Here's how the part is built. I have some questions about the finished solid (model axes, mm). A direction names the side the tool comes from. Round coordinates to 2 decimals unless told otherwise and drop trailing zeros. Write each loop counter-clockwise with the first axis right and the second up, starting at its lowest first coordinate (ties: lowest second). Pieces come first, ordered by that corner, then holes. Notation, with made-up numbers: (22.5, 2) - (45.5, 2) arc R35 cw to (45.5, 34) - close; hole circle Ø7 at (-6, 67). An arc over 180 degrees is marked (long way). Write item = value, one per line. Start each with the question number.
Item 1: Thinking about a two-plate mould opening in Y: for faces 3 (the face through (58.681, 294, 1)), 4 (the face through (21, 295.136, 1)), 5 (the face through (7.682, 293.538, 1.479)), 6 (the face through (35, 294, 0)), which applies, pulls with the +Y half, pulls with the -Y half, needs draft (parallel to the pull), parting line crosses it, or undercut?
Item 2: If we section it at B-B (z = 2.45): Please give me the cut outline in (x, y).
Item 3: If we section it at A-A (y = 294): Please give me the cut outline in (x, z), and give its area (3 significant figures).
Item 4: Which directions (+Z, -Z, +X, -X, +Y, -Y) give clear straight access to the entire face, cutting with the end or side of a thin tool? Please do faces 1 (the face through (35, 294, 3)), 2 (the face through (19.681, 294, 1)).
Item 5: If we section it at C-C (x = 58): Please give me the cut outline in (y, z).
Item 6: If we section it at D-D (y = 296): Please give me the cut outline in (x, z).
Item 7: If I drill on line 1 along Y through (x, z) = (29, 1.7); line 2 along Y through (x, z) = (58.5, 2.8); line 3 along Y through (x, z) = (10, 1.6), over which ranges is the centre line in solid material (lowest first)? Write a range as [from, to].
Item 8: For P1, Ø1, axis at y = 293, z = 1, coming from the +X side, with a flat end and sliding along its axis, tell me the tip position at first contact or that it passes through.
```python
from build123d import *

# Parameters (mm, degrees)
MODEL_W                 = 3
MODEL_H                 = 3
SALIENTE_EXTRUIR1_DEPTH = 3


with BuildPart() as part:
    # Model → Saliente-Extruir1 (new body)
    with BuildSketch(Plane.XY):
        with BuildLine():
            Line((12.181222481, 298.136475095), (57.181222481, 298.136475095))
            ThreePointArc((57.181222481, 298.136475095), (61.681222481, 293.636475095), (57.181222481, 289.136475095))
            Line((57.181222481, 289.136475095), (12.181222481, 289.136475095))
            ThreePointArc((12.181222481, 289.136475095), (7.681222481, 293.636475095), (12.181222481, 298.136475095))
        make_face()
        with Locations((12.181222481, 293.636475095)):
            Rectangle(MODEL_W, MODEL_H, mode=Mode.SUBTRACT)
        with Locations((21.181222481, 293.636475095)):
            Rectangle(MODEL_W, MODEL_H, mode=Mode.SUBTRACT)
        with Locations((30.181222481, 293.636475095)):
            Rectangle(MODEL_W, MODEL_H, mode=Mode.SUBTRACT)
        with Locations((39.181222481, 293.636475095)):
            Rectangle(MODEL_W, MODEL_H, mode=Mode.SUBTRACT)
        with Locations((57.181222481, 293.636475095)):
            Rectangle(MODEL_W, MODEL_H, mode=Mode.SUBTRACT)
        with Locations((48.181222481, 293.636475095)):
            Rectangle(MODEL_W, MODEL_H, mode=Mode.SUBTRACT)
    extrude(amount=SALIENTE_EXTRUIR1_DEPTH)


solid = part.part
```
Reply:
q1.face_3 = undercut
q1.face_4 = undercut
q1.face_5 = parting line crosses it
q1.face_6 = needs draft
q2.outline = (12.18, 289.14) - (57.18, 289.14) arc R4.5 ccw to (57.18, 298.14) - (12.18, 298.14) arc R4.5 ccw to start; hole (10.68, 292.14) - (13.68, 292.14) - (13.68, 295.14) - (10.68, 295.14) - close; hole (19.68, 292.14) - (22.68, 292.14) - (22.68, 295.14) - (19.68, 295.14) - close; hole (28.68, 292.14) - (31.68, 292.14) - (31.68, 295.14) - (28.68, 295.14) - close; hole (37.68, 292.14) - (40.68, 292.14) - (40.68, 295.14) - (37.68, 295.14) - close; hole (46.68, 292.14) - (49.68, 292.14) - (49.68, 295.14) - (46.68, 295.14) - close; hole (55.68, 292.14) - (58.68, 292.14) - (58.68, 295.14) - (55.68, 295.14) - close
q3.outline = (7.7, 0) - (10.68, 0) - (10.68, 3) - (7.7, 3) - close; (13.68, 0) - (19.68, 0) - (19.68, 3) - (13.68, 3) - close; (22.68, 0) - (28.68, 0) - (28.68, 3) - (22.68, 3) - close; (31.68, 0) - (37.68, 0) - (37.68, 3) - (31.68, 3) - close; (40.68, 0) - (46.68, 0) - (46.68, 3) - (40.68, 3) - close; (49.68, 0) - (55.68, 0) - (55.68, 3) - (49.68, 3) - close; (58.68, 0) - (61.67, 0) - (61.67, 3) - (58.68, 3) - close
q3.area = 108 mm2
q4.face_1 = +Z, +X, -X, +Y, -Y
q4.face_2 = +Z, -Z
q5.outline = (289.21, 0) - (292.14, 0) - (292.14, 3) - (289.21, 3) - close; (295.14, 0) - (298.06, 0) - (298.06, 3) - (295.14, 3) - close
q6.outline = (8.35, 0) - (61.01, 0) - (61.01, 3) - (8.35, 3) - close
q7.line_1 = [289.14, 292.14], [295.14, 298.14]
q7.line_2 = [289.33, 292.14], [295.14, 297.94]
q7.line_3 = [289.7, 297.57]
q8.P1 = 61.68
